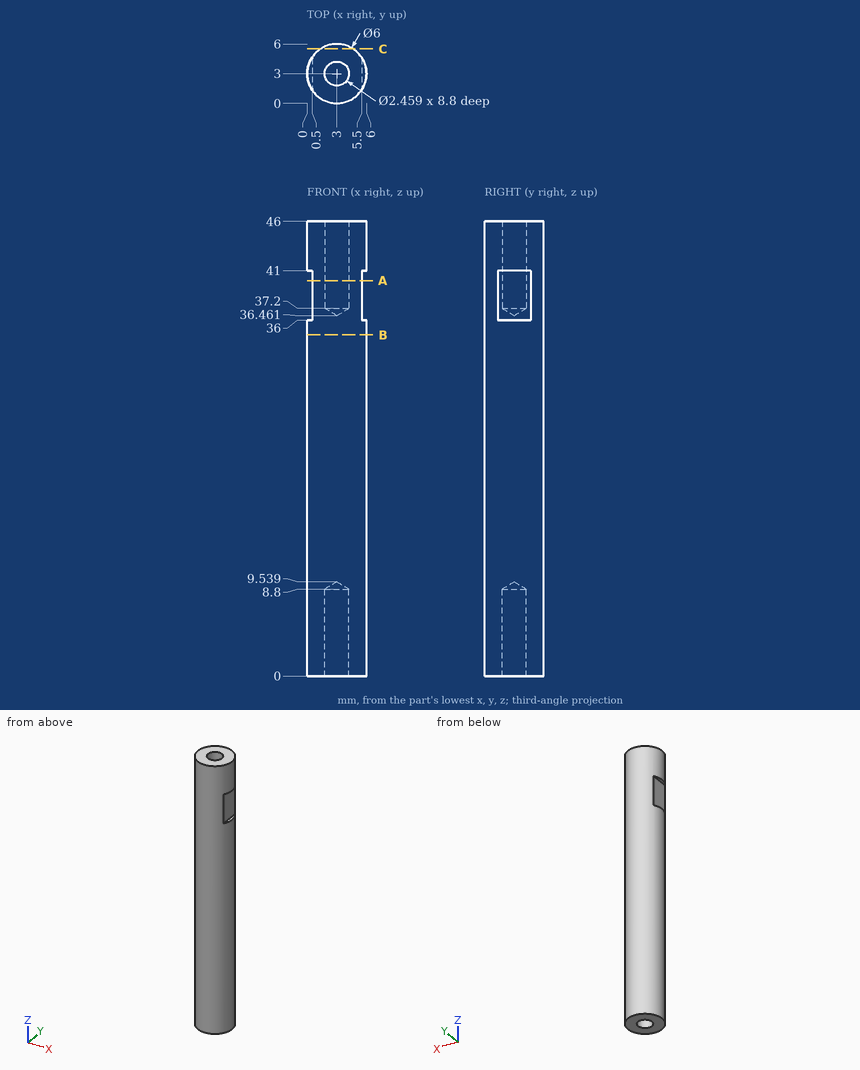
Verification items for this drawing (mm, ordinates from the low corner). Coordinates: 2 decimals unless noted, no trailing zeros. Order: outer loops, then holes, each group sorted by start corner. A loop starts at its lowest first (then second) coordinate and runs counter-clockwise, first axis right, second up. Notation, with made-up numbers: (22.5, 73) -> (30.5, 73) arc R18 cw to (30.5, 96) -> close; hole circle Ø8 at (17.5, -28.75). An arc over 180 degrees is marked (long way). Put each result on its own line as item: value. Start each with the question number.
1. Cross-section at A-A, the plane z = 40. Record the boundary of the cut face in (x, y), then the cut area to 3 significant figures.
2. Cross-section at C-C, the plane y = 5.5. Record the boundary of the cut face in (x, z), then the cut area to 3 significant figures.
3. Cross-section at B-B, the plane z = 34.5. Record the boundary of the cut face in (x, y).
4. Material ranges on L1, parallel to X at y = 3, z = 6.75; L2, parallel to Z at x = 0.45, y = 4.3; L3, parallel to X at y = 3.05, z = 39, recorded low to high. Write a range as [from, to].
5. Go/stop test with flat-tipped pins: pin 1 Ø3.5 at (y, z) = (3, 38) entering from -X; pin 2 Ø1 at (x, z) = (5, 13) entering from +Y. Record where each tip stops, or that it passes through.
Computed:
1. outline: (0.5, 1.34) arc R3 ccw to (5.5, 1.34) -> (5.5, 4.66) arc R3 ccw to (0.5, 4.66) -> close; hole circle Ø2.46 at (3, 3)
1. area: 21.3 mm2
2. outline: (1.34, 0) -> (4.66, 0) -> (4.66, 46) -> (1.34, 46) -> close
2. area: 153 mm2
3. outline: circle Ø6 at (3, 3)
4. L1: [0, 1.77], [4.23, 6]
4. L2: [0, 36], [41, 46]
4. L3: [0.5, 1.77], [4.23, 5.5]
5. pin 1: x = 0.5
5. pin 2: y = 5.6
